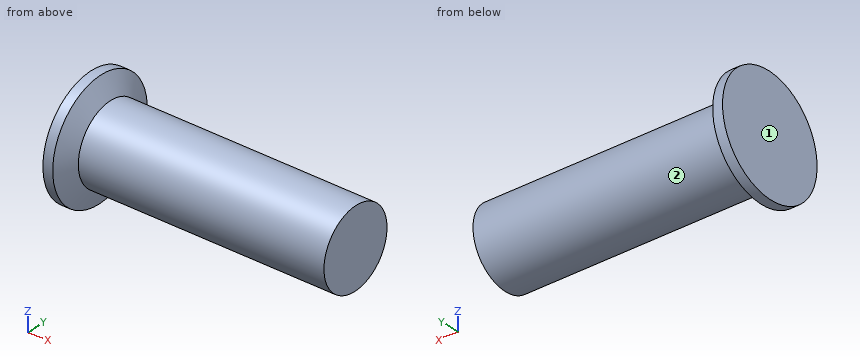
```python
from build123d import *

# Parameters (mm, degrees)
SKETCH1_R           = 3
BOSS_EXTRUDE1_DEPTH = 1
SKETCH1_4_R         = 2
BOSS_EXTRUDE2_DEPTH = 13.5


with BuildPart() as part:
    # Sketch1 → Boss-Extrude1 (new body)
    with BuildSketch(Plane.YZ):
        with Locations(Location((0, 0, 0), (0, 0, 270))):
            Circle(SKETCH1_R)
    extrude(amount=BOSS_EXTRUDE1_DEPTH)

    # Sketch1_4 → Boss-Extrude2 (add)
    with BuildSketch(Plane.YZ):
        with Locations(Location((0, 0, 0), (0, 0, 270))):
            Circle(SKETCH1_4_R)
    extrude(amount=BOSS_EXTRUDE2_DEPTH)

    # Sketch2 → Cut-Revolve1 (revolve, cut)
    with BuildSketch(Plane(origin=(0, 0, 0), x_dir=(-1, 0, 0), z_dir=(0, 1, 0)), mode=Mode.PRIVATE) as cut_revolve1_sk:
        Polygon((-0.5, 3), (-1, 2), (-1, 3), align=None)
    revolve(cut_revolve1_sk.sketch.rotate(Axis((0.683677116, 0, 0), (-1, 0, 0)), 180), axis=Axis((0.683677116, 0, 0), (-1, 0, 0)), mode=Mode.SUBTRACT)


solid = part.part
```
Input: part model. Units: mm. Frame: model coordinates. Face numbers are marked on the shaded views. A direction names the side the tool comes from. Round coordinates to 2 decimals unless told otherwise and drop trailing zeros. Loops run counter-clockwise (first coordinate to the right, second up) from the corner with the lowest first, then second, coordinate; pieces in that order, holes last. Notation, with made-up numbers: (66, -30) - (76, -30) arc R23 cw to (76, -10) - close; hole circle Ø9 at (-10, -37). An arc over 180 degrees is marked (long way). One line per item, written item: value. Start each with the question number.
(1) Section A-A, the plane z = 0. Return loops of the section in (x, y).
(2) Ray query, line 1 (Y direction, x = 7.25, z = 0.1); line 2 (Y direction, x = 9.75, z = 1.75); line 3 (Z direction, x = 3.5, y = -0.5). Return the intervals inside material, ascending. Write a range as [from, to].
(3) Access query for the marked faces 1 and 2. Directions: +Z, -Z, +X, -X, +Y, -Y. A direction counts if a zero-diameter tool reaches every point of the face in a straight line with its end or side. Return the directions, or none.
(4) Contact query for flat-ended pins moving along their axis: P1, Ø1.5, axis at x = 10, z = -2, coming from the -Y side; P2, Ø2, axis at x = 3, y = -0.5, coming from the -Z side; P3, Ø1, axis at x = 6, y = -0.5, coming from the +Z side. Output: stop coordinate, or through.
(5) Section C-C, the plane x = 3.75. Return loops of the section in (y, z).
Results below:
1. outline: (0, -3) - (0.5, -3) - (1, -2) - (13.5, -2) - (13.5, 2) - (1, 2) - (0.5, 3) - (0, 3) - close
2. line 1: [-2, 2]
2. line 2: [-0.97, 0.97]
2. line 3: [-1.94, 1.94]
3. face 1: +Z, -Z, -X, +Y, -Y
3. face 2: +X
4. P1: y = -1.56
4. P2: z = -2
4. P3: z = 2
5. outline: circle Ø4 at (0, 0)
